```python
from build123d import *

# Parameters (mm, degrees)
F0_W     = 270
F0_H     = 90
F0_R     = 2
F1_DEPTH = 0.635
F2_W     = 30
F2_H     = 40
F2_W_2   = 25.4
F2_H_2   = 60
F3_DEPTH = 0.636


with BuildPart() as f1:
    # F0 (on Top) → F1 (new body)
    with BuildSketch(Plane.XY):
        with Locations((135, -45)):
            Rectangle(F0_W, F0_H)
        with Locations((3.175, -80)):
            Circle(F0_R, mode=Mode.SUBTRACT)
        with Locations((40, -68)):
            Circle(F0_R, mode=Mode.SUBTRACT)
        with Locations((116.825, -84)):
            Circle(F0_R, mode=Mode.SUBTRACT)
        with Locations((40, -52)):
            Circle(F0_R, mode=Mode.SUBTRACT)
        with Locations((153.175, -84)):
            Circle(F0_R, mode=Mode.SUBTRACT)
        with Locations((266.825, -80)):
            Circle(F0_R, mode=Mode.SUBTRACT)
        with Locations((230, -68)):
            Circle(F0_R, mode=Mode.SUBTRACT)
        with Locations((230, -52)):
            Circle(F0_R, mode=Mode.SUBTRACT)
        with Locations((3.175, -10)):
            Circle(F0_R, mode=Mode.SUBTRACT)
        with Locations((105, -10)):
            Circle(F0_R, mode=Mode.SUBTRACT)
        with Locations((116.825, -9)):
            Circle(F0_R, mode=Mode.SUBTRACT)
        with Locations((153.175, -9)):
            Circle(F0_R, mode=Mode.SUBTRACT)
        with Locations((165, -10)):
            Circle(F0_R, mode=Mode.SUBTRACT)
        with Locations((266.825, -10)):
            Circle(F0_R, mode=Mode.SUBTRACT)
    extrude(amount=F1_DEPTH)

    # F2 (on face) → F3 (cut, through all)
    with BuildSketch(Plane.XY.offset(0.635)):
        with Locations((135, -20)):
            Rectangle(F2_W, F2_H)
        with Locations((24.125, -60)):
            Rectangle(F2_W_2, F2_H_2)
        with Locations((245.875, -60)):
            Rectangle(F2_W_2, F2_H_2)
    extrude(amount=-F3_DEPTH, mode=Mode.SUBTRACT)


solid = f1.part
```
Build history of the part. All positions in model axes, mm. Coordinates: 2 decimals unless noted, no trailing zeros. Write each loop counter-clockwise with the first axis right and the second up, starting at its lowest first coordinate (ties: lowest second). Pieces come first, ordered by that corner, then holes.
1. Band-saw the part on A-A, the plane y = -24.5. Give the cut face in (x, z) (3 decimals), and give its area (3 significant figures).
Answer block:
outline: (0, 0) - (120, 0) - (120, 0.635) - (0, 0.635) - close; (150, 0) - (270, 0) - (270, 0.635) - (150, 0.635) - close
area: 152 mm2
2. Drill centre lines: probe 1 along X at (y, z) = (-77, 0.35) (3 decimals); probe 2 along X at (y, z) = (-53, 0.2) (3 decimals); probe 3 along Y at (x, z) = (28.5, 0.6). Where is each one in solid material? Low to high.
Answer block:
probe 1: x = 0 to 11.425, 36.825 to 233.175, 258.575 to 270
probe 2: x = 0 to 11.425, 36.825 to 38.268, 41.732 to 228.268, 231.732 to 233.175, 258.575 to 270
probe 3: y = -30 to 0
3. Band-saw the part on B-B, the plane y = -57. Give the cut face in (x, z) (3 decimals), and give its area (3 significant figures).
Answer block:
outline: (0, 0) - (11.425, 0) - (11.425, 0.635) - (0, 0.635) - close; (36.825, 0) - (233.175, 0) - (233.175, 0.635) - (36.825, 0.635) - close; (258.575, 0) - (270, 0) - (270, 0.635) - (258.575, 0.635) - close
area: 139 mm2
4. Band-saw the part on C-C, the plane z = 0.5. Give the number of separate pieces and of enclosed holes in the cut face, and give its area (3 significant figures).
Answer block:
separate pieces: 1
enclosed holes: 14
area: 19,900 mm2
